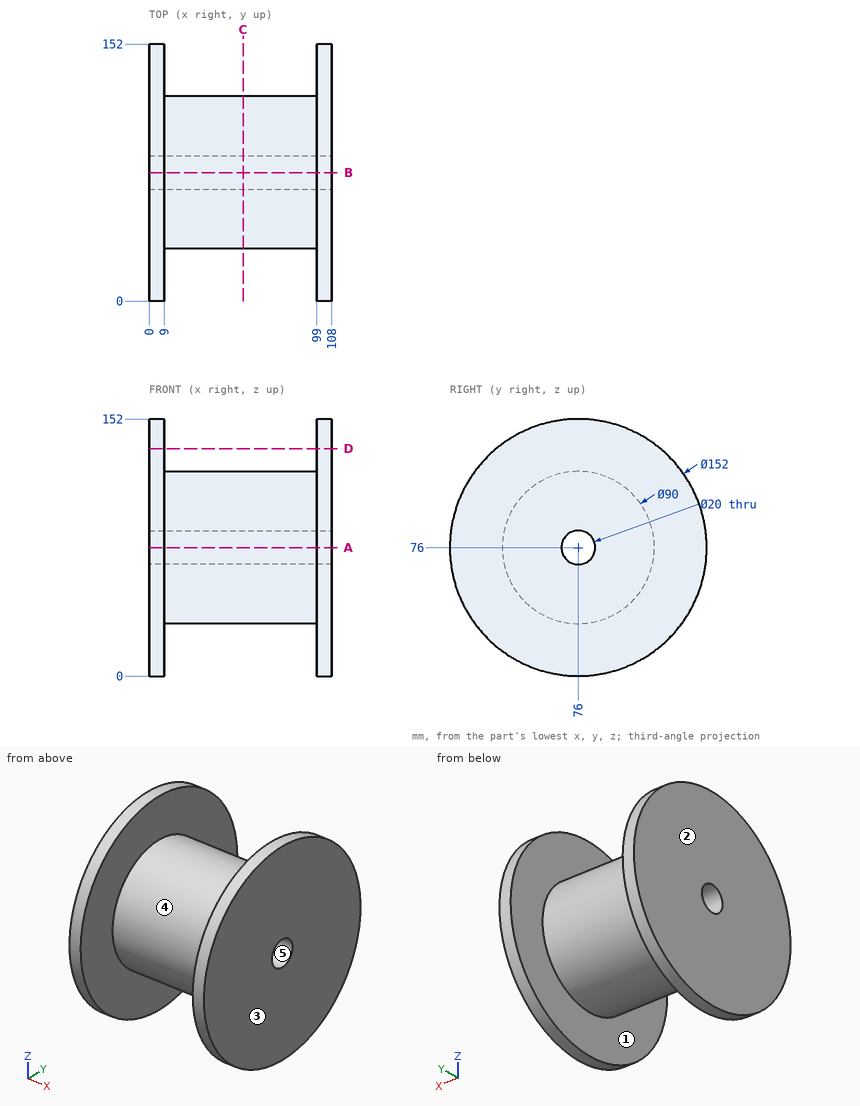
For this review, use the dimensioned drawing (mm, ordinates from the lowest corner) and the shaded views. A direction names the side the tool comes from. Give positions to 0.01 mm unless a question says otherwise; leave off trailing zeros. Order: outer loops, then holes, each group sorted by start corner. A loop starts at its lowest first (then second) coordinate and runs counter-clockwise, first axis right, second up. Notation, with made-up numbers: (56, -29.5) - (104, -29.5) arc R38 cw to (104, 9.5) - close; hole circle Ø9 at (44.5, -18.5). An arc over 180 degrees is marked (long way). Use a Markdown table: item, result. Add a question column.
(1) Mouldability with a two-part tool opening along Y and no side actions: class the marked faces 3, 4 and 5 as +Y half, -Y half, draft (parallel to the pull), parting line (faces both ways), or undercut.
(2) Wall thickness on probe 1 along Y at (x, z) = (61.5, 76); probe 2 along X at (y, z) = (21.5, 123); probe 3 along Z at (x, y) = (44.5, 76.5): over which ranges is each line inside the solid? List them lowest first. Write a range as [from, to].
(3) Add section A-A on z = 76. Give the boundary of the cut face in (x, y), then the cut area to 3 significant figures.
(4) Add section D-D on z = 134.5. Give the boundary of the cut face in (x, y).
(5) Machinability: for the marked faces 1 and 2, which of the approach directions +Z, -Z, +X, -X, +Y, -Y give a long, thin tool a straight path to every point of the face, cutting with its end or side? Answer none if there is none.
(6) Add section C-C on x = 55.5. Give the boundary of the cut face in (y, z).
(7) Clearance check with flat-ended pins moving along their axes: P1, Ø6, axis at x = 80.5, z = 110.5, coming from the +Y side; P2, Ø8, axis at x = 67, y = 93, coming from the -Z side; P3, Ø12, axis at x = 55.5, z = 85, coming from the +Y side. State where each tip first meets the part, or that it passes through.
Report:
| question | item | result |
|---|---|---|
| 1 | face 3 | draft |
| 1 | face 4 | parting line |
| 1 | face 5 | undercut |
| 2 | probe 1 | y = [31, 66], [86, 121] |
| 2 | probe 2 | x = [0, 9], [99, 108] |
| 2 | probe 3 | z = [31, 66.01], [85.99, 121] |
| 3 | outline | (0, 0) - (9, 0) - (9, 31) - (99, 31) - (99, 0) - (108, 0) - (108, 66) - (0, 66) - close; (0, 86) - (108, 86) - (108, 152) - (99, 152) - (99, 121) - (9, 121) - (9, 152) - (0, 152) - close |
| 3 | area | 8,680 mm² |
| 4 | outline | (0, 27.48) - (9, 27.48) - (9, 124.52) - (0, 124.52) - close; (99, 27.48) - (108, 27.48) - (108, 124.52) - (99, 124.52) - close |
| 5 | face 1 | none |
| 5 | face 2 | +Z, -Z, -X, +Y, -Y |
| 6 | outline | circle Ø90 at (76, 76); hole circle Ø20 at (76, 76) |
| 7 | P1 | stops at y = 108.14 |
| 7 | P2 | stops at z = 32.92 |
| 7 | P3 | stops at y = 120.9 |
